Verification items for the finished model (mm, model axes). A direction names the side the tool comes from. Coordinates: 2 decimals unless noted, no trailing zeros. Write each loop counter-clockwise with the first axis right and the second up, starting at its lowest first coordinate (ties: lowest second). Pieces come first, ordered by that corner, then holes. Notation, with made-up numbers: (79.25, 21.5) -> (109.25, 21.5) arc R7 cw to (109.25, 32.5) -> close; hole circle Ø4 at (72, -23). An arc over 180 degrees is marked (long way). Use CSV: the item, a comma, the result in double quotes.
Autodesk Inventor part; units mm, degrees
ref_plane "YZ Plane" through (0, 0, 0) normal (1, 0, 0) x (0, 1, 0)
ref_plane "XZ Plane" through (0, 0, 0) normal (0, 1, 0) x (-1, 0, 0)
ref_plane "XY Plane" through (0, 0, 0) normal (0, 0, 1) x (1, 0, 0)
sketch "Sketch1" plane through (0, 0, 0) normal (0, 0, 1) x (1, 0, 0)
  circle A0 centre (0, 0) radius 2
  dimension "Diameter" = 4
extrude "Extrusion1" add sketch "Sketch1" along normal blind 9.52
sketch "Sketch2" plane through (0, 0, 9.52) normal (0, 0, 1) x (1, 0, 0)
  circle A0 centre (0, 0) radius 2
extrude "Extrusion2" add sketch "Sketch2" along normal blind 2.48 draft 45
sketch "Sketch3" plane through (0, 0, 12) normal (0, 0, 1) x (1, 0, 0)
  circle A0 centre (0, 0) radius 4.48
  circle A1 centre (0, 0) radius 1.4434 construction
  line L0 (0.6042, 1.3108) -> (1.4373, 0.1322)
  line L1 (1.4373, 0.1322) -> (0.8331, -1.1787)
  line L2 (0.8331, -1.1787) -> (-0.6042, -1.3108)
  line L3 (-0.6042, -1.3108) -> (-1.4373, -0.1322)
  line L4 (-1.4373, -0.1322) -> (-0.8331, 1.1787)
  line L5 (-0.8331, 1.1787) -> (0.6042, 1.3108)
  dimension "Hex_Width" = 2.5
extrude "Extrusion3" cut sketch "Sketch3" against normal blind 1.5 contours L0 L1 L2 L3 L4 L5
thread "Thread1"
chamfer "Chamfer2" distance 0.4 angle 45 1 edges at (-2, 0, 0)
fillet "Fillet1" radius 0.1 1 edges at (-4.48, 0, 12)
equation "\"d13\" = Chamfer"
equation "\"Thread_Length\" = 7.52"
properties part number "SCREW, FLAT HD, P, 12_9, M4X0_7X12MM"
1) Cross-section at B-B (z = 9.75). Record the boundary of the cut face in (x, y), plus the area to 3 significant figures.
Return value:
outline,"circle Ø4.46 at (0, 0)"
area,"15.6 mm2"
2) Set-up check for faces 4 (the flat face through (-1.14, 0.51, 11.26)), 5 (the conical face through (2.045, 0.644, 9.664)): record each of +Z, -Z, +X, -X, +Y, -Y from which the full face is reachable in a straight line by a thin tool's end or side.
Return value:
face 4,"+Z"
face 5,"-Z"
3) Scan lines: L1, parallel to Z at x = 0.5, y = -0.5; L2, parallel to Y at x = -0.75, z = 11; L3, parallel to X at y = -1, z = 7.75. Record each from-to range of solid material in increasing order.
Return value:
L1,"0 to 10.5"
L2,"-3.4 to -1.1, 1.19 to 3.4"
L3,"-1.73 to 1.73"
4) Gauge pin test, flat ends, axial feed: pin 1 (4 mm diameter, centred on x = -1, z = 8, fed in from -Y); pin 2 (4 mm diameter, centred on y = -2, z = 5, fed in from +X); pin 3 (1 mm diameter, centred on y = 1.5, z = 1.5, fed in from -X). Record the tip position at first contact, or that the pin passes through.
Return value:
pin 1,"y = -2.37"
pin 2,"x = 2"
pin 3,"x = -1.73"
5) Cross-section at C-C (x = 0). Record the boundary of the cut face in (y, z), plus the area to 3 significant figures.
Return value:
outline,"(-4.31, 11.83) -> (-2, 9.52) -> (-2, 0.4) -> (-1.6, 0) -> (1.6, 0) -> (2, 0.4) -> (2, 9.52) -> (4.31, 11.83) arc R0.1 ccw to (4.24, 12) -> (1.26, 12) -> (1.26, 10.5) -> (-1.26, 10.5) -> (-1.26, 12) -> (-4.24, 12) arc R0.1 ccw to start"
area,"50.2 mm2"
6) Mould release check, pull along Y, two halves, no side actions. Record for faces 1 (the cylindrical face through (0, 2, 5)), 2 (the flat face through (0, 0, 0)), 3 (the flat face through (0.125, -1.244, 11.26)): released by +Y, released by -Y, zero draft, split by the parting line, or undercut.
Return value:
face 1,"split by the parting line"
face 2,"zero draft"
face 3,"undercut"
7) Cross-section at D-D (z = 5.5). Record the boundary of the cut face in (x, y).
Return value:
outline,"circle Ø4 at (0, 0)"
8) Cross-section at A-A (z = 11). Record the boundary of the cut face in (x, y), plus the area to 3 significant figures.
Return value:
outline,"circle Ø6.96 at (0, 0); hole (-1.44, -0.13) -> (-0.6, -1.31) -> (0.83, -1.18) -> (1.44, 0.13) -> (0.6, 1.31) -> (-0.83, 1.18) -> close"
area,"32.6 mm2"
